```python
from build123d import *

# Parameters (mm, degrees)
F3_DEPTH = 15.24


with BuildPart() as f1:
    # F0 (on Top) → F1 (revolve)
    with BuildSketch(Plane.XY):
        with BuildLine():
            ThreePointArc((-1.032711, 0), (-0.880739, 2.768468), (0, 5.3975))
            Line((0, 5.3975), (-2.286, 5.3975))
            ThreePointArc((-2.286, 5.3975), (-8.654858, 3.331535), (-15.24, 2.120558))
            Line((-15.24, 2.120558), (-45.731511, 2.120558))
            Line((-45.731511, 2.120558), (-50.811511, 0))
            Line((-50.811511, 0), (-1.032711, 0))
        make_face()
    revolve(axis=Axis((-25.922111, 0, 0), (-1, 0, 0)))

    # F2 (on Right) → F3 (cut)
    with BuildSketch(Plane.YZ):
        Polygon((3.833906, -5.929406), (0, -2.0955), (-3.833906, -5.929406), align=None)
        Polygon((-6.421372, -4.325872), (-2.0955, 0), (-6.421372, 4.325872), align=None)
        Polygon((6.06417, 3.96867), (2.0955, 0), (6.06417, -3.96867), align=None)
        Polygon((-4.487521, 6.583021), (0, 2.0955), (4.487521, 6.583021), align=None)
    extrude(amount=-F3_DEPTH, mode=Mode.SUBTRACT)


solid = f1.part
```
Part model, mm, in its own coordinate system. A direction names the side the tool comes from. Coordinates: 2 decimals unless noted, no trailing zeros. Write each loop counter-clockwise with the first axis right and the second up, starting at its lowest first coordinate (ties: lowest second). Pieces come first, ordered by that corner, then holes.
Item 1: Mould opens along Z. For faces 1 (the face through (-48.87, -0.18, 0.79)), 2 (the face through (-4.127, -3.134, -1.038)), 3 (the face through (-5.82, -1.001, -3.097)) say: released by +Z, released by -Z, zero draft, split by the parting line, or undercut.
Item 2: Probe line 1 (Z direction, x = -7.5, y = 3); line 2 (Y direction, x = -8, z = 2.75); line 3 (Y direction, x = -3.5, z = 3). List the from-to ranges inside material, lowest first.
Item 3: Which spindle directions (+Z, -Z, +X, -X, +Y, -Y) get a long thin tool onto all of the face, cutting with end or side? Do faces 4 (the face through (-1.159, 3.831, -3.802)), 5 (the face through (-30.7, -0.46, 2.07)). Say none if no direction does.
Item 4: Pin check, flat tips, straight feed: pin 1 (5 mm diameter, centred on y = 0, z = 0.5, fed in from -X); pin 2 (1 mm diameter, centred on y = 3.5, z = 2, fed in from +X); pin 3 (3 mm diameter, centred on x = -30.5, y = 1, fed in from +Z); pin 4 (2 mm diameter, centred on x = -30, y = -0.5, fed in from -Z). Stop position of each tip, or through.
Item 5: Slice it at A-A (x = -11.5). Write the cut outline in (y, z), and give its area (3 significant figures).
Item 6: Slice it at B-B (x = -23). Write the cut outline in (y, z).
Results found:
1. face 1: split by the parting line
1. face 2: undercut
1. face 3: released by -Z
2. line 1: z = -2.06 to -0.9, 0.9 to 2.06
2. line 2: y = -2.17 to -0.65, 0.65 to 2.17
2. line 3: y = -3.91 to -0.9, 0.9 to 3.91
3. face 4: -Z, +X, -X, +Y
3. face 5: -X
4. pin 1: stops at x = -50.81
4. pin 2: stops at x = -0.38
4. pin 3: stops at z = 2.12
4. pin 4: stops at z = -2.12
5. outline: (-2.64, -0.55) arc R2.7 ccw to (-0.55, -2.64) - (0, -2.1) - (0.55, -2.64) arc R2.7 ccw to (2.64, -0.55) - (2.1, 0) - (2.64, 0.55) arc R2.7 ccw to (0.55, 2.64) - (0, 2.1) - (-0.55, 2.64) arc R2.7 ccw to (-2.64, 0.55) - (-2.1, 0) - close
5. area: 21.5 mm2
6. outline: circle Ø4.24 at (0, 0)
